Answer from the drawing. Dimensions are ordinates in mm from the lowest x, y and z of the part. Give positions to 0.01 mm unless a question says otherwise; leave off trailing zeros. Write each loop counter-clockwise with the first axis right and the second up, starting at its lowest first coordinate (ties: lowest second). Pieces come first, ordered by that corner, then holes. Notation, with made-up numbers: (3, 37.5) -> (36, 37.5) arc R11 cw to (36, 52.5) -> close; hole circle Ø7 at (52, -38). An arc over 180 degrees is marked (long way). Put each result on its own line as item: value. Start each with the question number.
1) A cutting plane is placed at A-A (y = 45). Write down the section's boundary in (x, z), then the cut area to 3 significant figures.
2) A flat-ended cylindrical pin translates along its axis: pin 1 Ø1.8 at (x, y) = (26, 45) entering from +Z. Find the tip coordinate at first contact, or state that the pin passes through.
3) Find the intervals of material crossed by line 1 along Y through (x, z) = (3, 0.55); line 2 along X through (y, z) = (45, 0.2); line 3 along Y through (x, z) = (2.5, 0.5), in increasing order. Write a range as from..to.
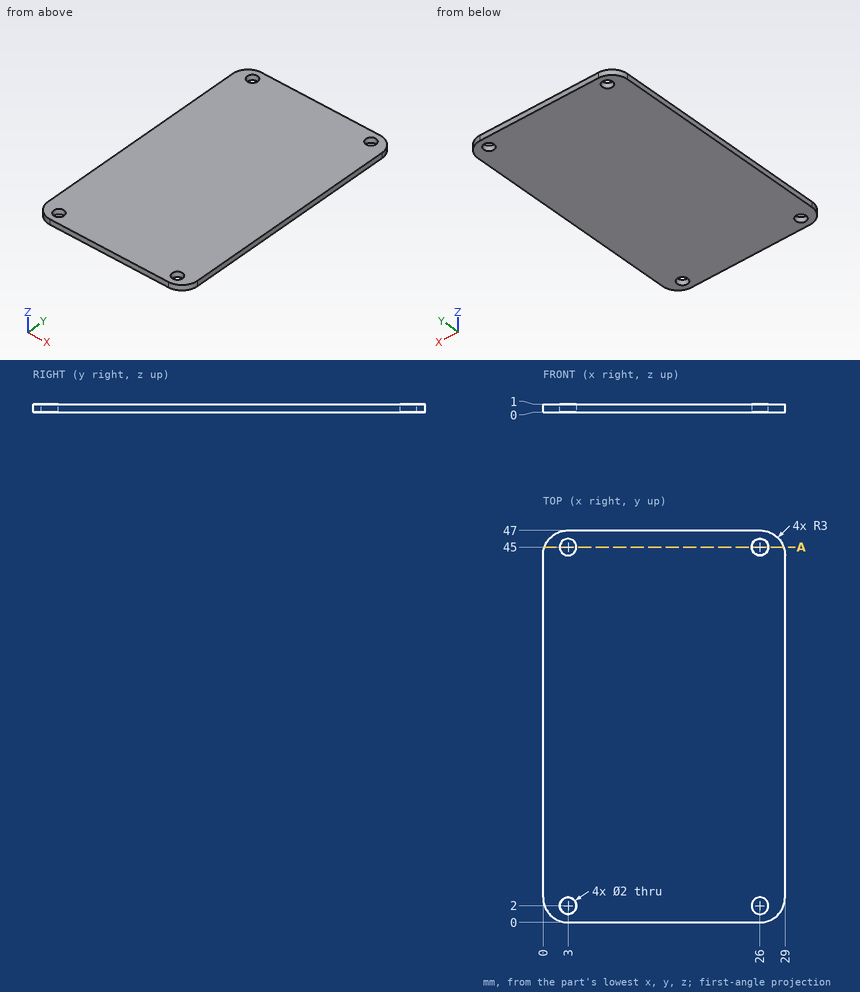
Reply:
1. outline: (0.17, 0) -> (2, 0) -> (2, 1) -> (0.17, 1) -> close; (4, 0) -> (25, 0) -> (25, 1) -> (4, 1) -> close; (27, 0) -> (28.83, 0) -> (28.83, 1) -> (27, 1) -> close
1. area: 24.7 mm2
2. pin 1: passes through
3. line 1: y = 0..1, 3..44, 46..47
3. line 2: x = 0.17..2, 4..25, 27..28.83
3. line 3: y = 0.04..1.13, 2.87..44.13, 45.87..46.96
